from build123d import *

# Parameters (mm, degrees)
F0_R     = 19.950599
F0_R_2   = 11.920368
F1_DEPTH = 38.1
F0_W     = 87.976367
F0_H     = 79.894547
F2_DEPTH = 25.4


with BuildPart() as f1:
    # F0 (on Top) → F1 (new body)
    with BuildSketch(Plane.XY):
        with Locations((4.849092, 2.193636)):
            Circle(F0_R)
        with Locations((4.849092, 2.193636)):
            Circle(F0_R_2, mode=Mode.SUBTRACT)
    extrude(amount=F1_DEPTH)

    # F0 (on Top) → F2 (join)
    with BuildSketch(Plane.XY):
        with Locations((6.35, -1.039089)):
            Rectangle(F0_W, F0_H)
        with Locations((4.849092, 2.193636)):
            Circle(F0_R, mode=Mode.SUBTRACT)
    extrude(amount=F2_DEPTH)


solid = f1.part
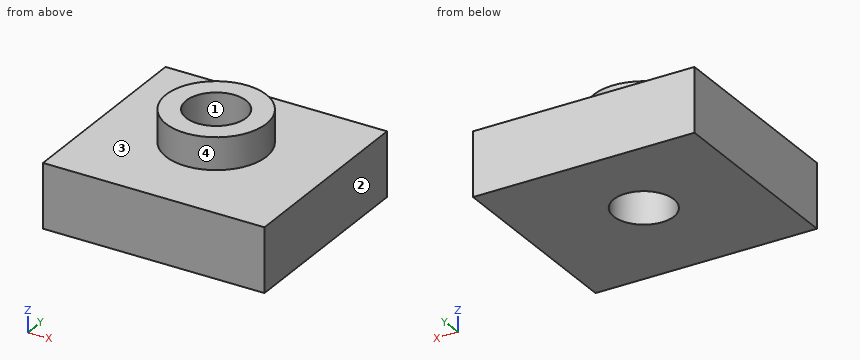
The listing builds one solid part. Answer for the finished solid, in the listing's coordinates (mm). Face numbers are marked on the shaded views. Round coordinates to 2 decimals unless told otherwise and drop trailing zeros. Write each loop counter-clockwise with the first axis right and the second up, starting at its lowest first coordinate (ties: lowest second). Pieces come first, ordered by that corner, then holes. Notation, with made-up numbers: M 73,57 L 97,57 A29 cw 97,88 Z; hole C -29.75,66 d10. An arc over 180 degrees is marked long. Write each question's results on one line, items separated by ' | '. Start each with the question number.
Item 1: A cutting plane is placed at B-B on x = 34.5. Write down the section's boundary in (y, z), and give its area (3 significant figures).
Item 2: Straight lines are drawn through the part: L1, parallel to Z at x = 12, y = -16.5; L2, parallel to Y at x = 5, z = 29.5; L3, parallel to Y at x = -5.5, z = 32.5. For each, find the intervals that lie inside material, in ascending order. Write a range as [from, to].
Item 3: A cutting plane is placed at C-C on z = 6.5. Write down the section's boundary in (x, y).
Item 4: For a pull along X with two mould halves and no side action, classify the marked faces 1, 2, 3 and 4 as pulls with the +X half, pulls with the -X half, needs draft (parallel to the pull), parting line crosses it, or undercut.
Item 5: A cutting plane is placed at D-D on y = -3.5. Write down the section's boundary in (x, z).
Item 6: A cutting plane is placed at A-A on y = 6.5. Write down the section's boundary in (x, z).
Item 7: Flat-ended cylindrical pins translate along their axes: pin 1 Ø14.5 at (x, y) = (4.85, 2.19) entering from -Z; pin 2 Ø10 at (y, z) = (1, 27) entering from -X; pin 3 Ø12 at (x, y) = (30, -27.5) entering from +Z. Find the tip coordinate at first contact, or state that the pin passes through.
Check sheet entries:
1) outline: M -40.99,0 L 38.91,0 L 38.91,25.4 L -40.99,25.4 Z | area: 2,030 mm²
2) L1: [0, 25.4] | L2: [-17.76, -9.73], [14.11, 22.14] | L3: [-14.86, -3.72], [8.11, 19.25]
3) outline: M -37.64,-40.99 L 50.34,-40.99 L 50.34,38.91 L -37.64,38.91 Z; hole C 4.85,2.19 d23.84
4) face 1: undercut | face 2: pulls with the +X half | face 3: needs draft | face 4: parting line crosses it
5) outline: M -37.64,0 L -5.62,0 L -5.62,38.1 L -14.27,38.1 L -14.27,25.4 L -37.64,25.4 Z; M 15.32,0 L 50.34,0 L 50.34,25.4 L 23.97,25.4 L 23.97,38.1 L 15.32,38.1 Z
6) outline: M -37.64,0 L -6.27,0 L -6.27,38.1 L -14.63,38.1 L -14.63,25.4 L -37.64,25.4 Z; M 15.96,0 L 50.34,0 L 50.34,25.4 L 24.33,25.4 L 24.33,38.1 L 15.96,38.1 Z
7) pin 1: through | pin 2: x = -37.64 | pin 3: z = 25.4
